Design review of the part shown in the three views and the two pictorial views. Dimensions are in mm from the part's minimum x, y and z. A direction names the side the tool comes from. Round coordinates to 2 decimals unless told otherwise and drop trailing zeros. Order: outer loops, then holes, each group sorted by start corner. A loop starts at its lowest first (then second) coordinate and runs counter-clockwise, first axis right, second up.
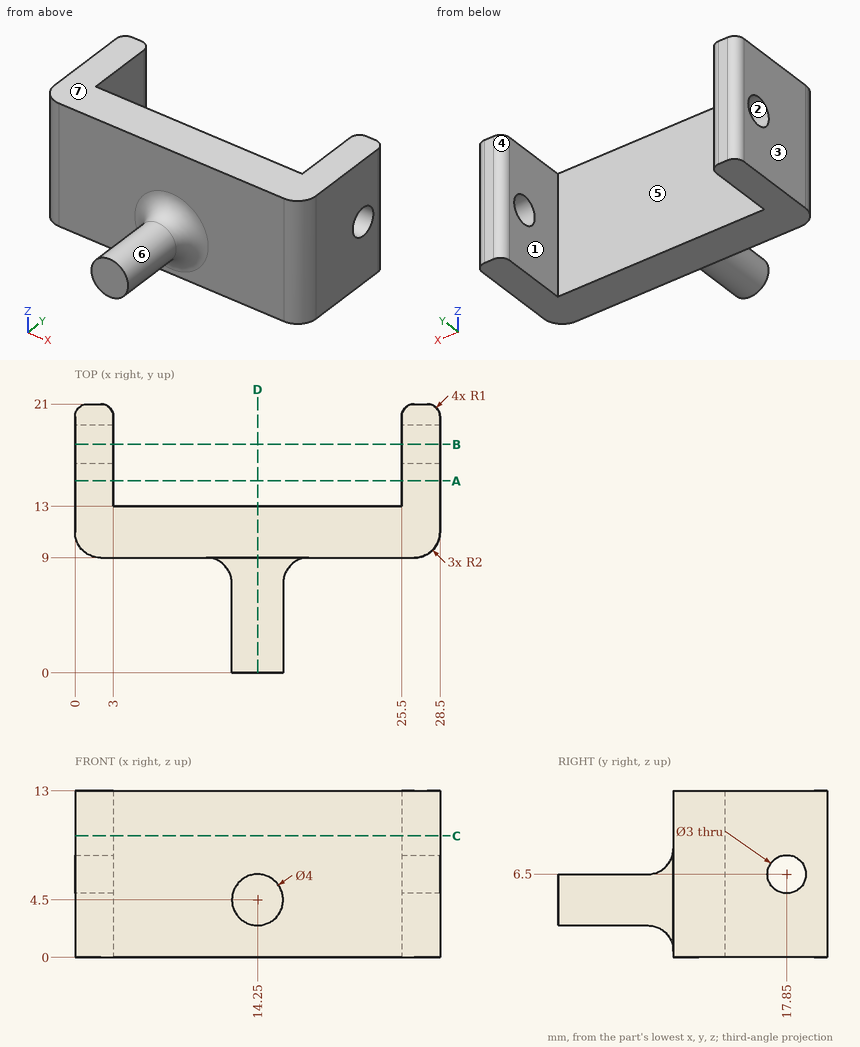
1) Take a section at D-D on x = 14.25. Give the boundary of the cut face in (y, z).
Results:
outline: (0, 2.5) - (7, 2.5) arc R2 cw to (9, 0.5) - (9, 0) - (13, 0) - (13, 13) - (9, 13) - (9, 8.5) arc R2 cw to (7, 6.5) - (0, 6.5) - close
2) Take a section at C-C on z = 9.5. Give the boundary of the cut face in (x, y), plus the area to 3 significant figures.
Results:
outline: (0, 11) arc R2 ccw to (2, 9) - (26.5, 9) arc R2 ccw to (28.5, 11) - (28.5, 20) arc R1 ccw to (27.5, 21) - (26.5, 21) arc R1 ccw to (25.5, 20) - (25.5, 13) - (3, 13) - (3, 20) arc R1 ccw to (2, 21) - (1, 21) arc R1 ccw to (0, 20) - close
area: 159 mm2
3) For the marked faces 5, 6 and 7, list the 3-axis set-ups (+Z, -Z, +X, -X, +Y, -Y) from which the entire face can be reached by the end or side of a thin tool; tool diameter is ignored.
Results:
face 5: +Z, -Z, +Y
face 6: -Y
face 7: +Z, +X, -X, +Y, -Y
4) Take a section at B-B on y = 17.85. Give the boundary of the cut face in (x, z), plus the area to 3 significant figures.
Results:
outline: (0, 0) - (3, 0) - (3, 5) - (0, 5) - close; (0, 8) - (3, 8) - (3, 13) - (0, 13) - close; (25.5, 0) - (28.5, 0) - (28.5, 5) - (25.5, 5) - close; (25.5, 8) - (28.5, 8) - (28.5, 13) - (25.5, 13) - close
area: 60.0 mm2
5) Clearance check with flat-ended pins moving along their axes: P1, Ø4, axis at x = 20, z = 9.5, coming from the +Y side; P2, Ø1.5, axis at x = 25, z = 6.5, coming from the +Y side; P3, Ø4, axis at y = 8, z = 6.5, coming from the -X side; P4, Ø2.5, axis at y = 17.85, z = 6.5, coming from the -X side. State where each tip first meets the part, or that it passes through.
Results:
P1: stops at y = 13
P2: stops at y = 20.66
P3: stops at x = 0.27
P4: passes through
6) The part is to be moulded in two halves that separate along X. For the marked faces 1, 2, 3 and 4, say which applies: released by +X, released by -X, zero draft, split by the parting line, or undercut.
Results:
face 1: undercut
face 2: zero draft
face 3: released by -X
face 4: undercut
7) Take a section at A-A on y = 15. Give the boundary of the cut face in (x, z).
Results:
outline: (0, 0) - (3, 0) - (3, 13) - (0, 13) - close; (25.5, 0) - (28.5, 0) - (28.5, 13) - (25.5, 13) - close
8) To check wall thickness, follow line 1 along X through (y, z) = (13.75, 10.5); line 2 along Y through (x, z) = (24.75, 6); line 3 along Y through (x, z) = (1.75, 6.5). State the ranges of each line that lie inside material, in increasing order.
Results:
line 1: x = 0 to 3, 25.5 to 28.5
line 2: y = 9 to 13
line 3: y = 9.02 to 16.35, 19.35 to 21
